Solid Edge part; units mm, degrees
sketch "Sketch1" plane through (0, 0, 0) normal (0, -1, 0) x (1, 0, 0)
  circle A0 centre (0, 0) radius 30
extrude "ExtrudedProtrusion_1" add sketch "Sketch1" against normal blind 700
sketch "Sketch2" plane through (0, 0, 0) normal (0, 0, 1) x (1, 0, 0)
  circle A0 centre (0, 700) radius 40
extrude "Protrusion1" add sketch "Sketch2" along normal mid plane 130
sketch "Sketch3" plane through (0, 528, 65) normal (0, 0, 1) x (1, 0, 0)
  circle A0 centre (0, 172) radius 30
extrude "Cutout1" cut sketch "Sketch3" against normal through all
Geometry check sheet. Reference: the model listing, model coordinates, mm. A direction names the side the tool comes from. Coordinates: 2 decimals unless noted, no trailing zeros. Loops run counter-clockwise (first coordinate to the right, second up) from the corner with the lowest first, then second, coordinate; pieces in that order, holes last. Notation, with made-up numbers: (12, 63) -> (57, 63) arc R11 cw to (57, 82) -> close; hole circle Ø11 at (34.25, 26). An arc over 180 degrees is marked (long way). Put each result on its own line as item: value.
1) Cross-section at C-C on z = 0. Record the boundary of the cut face in (x, y), plus the area to 3 significant figures.
Result set:
outline: (-30, 0) -> (30, 0) -> (30, 673.54) arc R40 ccw (long way) to (-30, 673.54) -> close; hole circle Ø60 at (0, 700)
area: 42,000 mm^2
2) Cross-section at B-B on x = 0. Record the boundary of the cut face in (y, z), plus the area to 3 significant figures.
Result set:
outline: (0, -30) -> (660, -30) -> (660, -65) -> (670, -65) -> (670, 65) -> (660, 65) -> (660, 30) -> (0, 30) -> close; (730, -65) -> (740, -65) -> (740, 65) -> (730, 65) -> close
area: 42,200 mm^2
3) Cross-section at A-A on y = 700. Record the boundary of the cut face in (x, z).
Result set:
outline: (-40, -65) -> (-30, -65) -> (-30, 65) -> (-40, 65) -> close; (30, -65) -> (40, -65) -> (40, 65) -> (30, 65) -> close
4) Tool access check on faces 4 (the cylindrical face through (-6.503, 332.056, -29.287)), 5 (the cylindrical face through (-8.67, 739.05, -0.91)), 6 (the flat face through (6, 730, -65)). Record the directions out of +Z, -Z, +X, -X, +Y, -Y that give a thin tool (end or side, any length) a straight path to the whole face; none if there is none.
Result set:
face 4: -Y
face 5: none
face 6: -Z, +X, -X, +Y, -Y
5) Cross-section at D-D on y = 458. Record the boundary of the cut face in (x, z).
Result set:
outline: circle Ø60 at (0, 0)
6) Gauge pin test, flat ends, axial feed: pin 1 Ø1.5 at (x, y) = (20.5, 197.5) entering from +Z; pin 2 Ø12 at (y, z) = (267, 12) entering from -X; pin 3 Ø3 at (x, z) = (-22, 35.5) entering from -Y. Record the tip position at first contact, or that the pin passes through.
Result set:
pin 1: stops at z = 22.58
pin 2: stops at x = -29.39
pin 3: stops at y = 665.65
7) Thickness scan on line 1 (Y direction, x = 0, z = -5.5); line 2 (Y direction, x = 0, z = -33); line 3 (X direction, y = 369, z = -2.5). Record the ranges inside material, lowest first.
Result set:
line 1: y = 0 to 670, 730 to 740
line 2: y = 660 to 670, 730 to 740
line 3: x = -29.9 to 29.9
8) Release check for a two-part mould opening along Y. For faces 1 (the flat face through (6, 730, 65)), 2 (the cylindrical face through (-3.905, 729.745, 0.91)), 3 (the flat face through (0, 0, 0)) record: released by +Y, released by -Y, zero draft, split by the parting line, or undercut.
Result set:
face 1: zero draft
face 2: undercut
face 3: released by -Y
